from build123d import *

# Parameters (mm, degrees)
SKETCH1_W                    = 126
SKETCH1_H                    = 130
SKETCH1_R                    = 32.5
SKETCH1_W_2                  = 4.9
SKETCH1_H_2                  = 20
BOSS_EXTRUDE1_DEPTH          = 3
SKETCH2_W                    = 2.9
SKETCH2_H                    = 20
CUT_EXTRUDE1_DEPTH           = 3
F_4_0_4_DIAMETER_HOLE1_D     = 4
F_4_0_4_DIAMETER_HOLE1_DEPTH = 10
F_4_0_4_DIAMETER_HOLE1_TIP   = 1.201721238
SKETCH6_R                    = 2.3
CUT_EXTRUDE2_DEPTH           = 3


with BuildPart() as part:
    # Sketch1 → Boss-Extrude1 (new body)
    with BuildSketch(Plane.XY):
        with Locations((0, -5)):
            Rectangle(SKETCH1_W, SKETCH1_H)
        Circle(SKETCH1_R, mode=Mode.SUBTRACT)
        with Locations((-17.5, -54.9)):
            Rectangle(SKETCH1_W_2, SKETCH1_H_2, mode=Mode.SUBTRACT)
        with Locations((17.5, -54.9)):
            Rectangle(SKETCH1_W_2, SKETCH1_H_2, mode=Mode.SUBTRACT)
    extrude(amount=BOSS_EXTRUDE1_DEPTH)

    # Sketch2 → Cut-Extrude1 (cut)
    with BuildSketch(Plane.XY.offset(3)):
        with Locations((-56.5, -0.4)):
            Rectangle(SKETCH2_W, SKETCH2_H)
    cut_extrude1 = extrude(amount=-CUT_EXTRUDE1_DEPTH, mode=Mode.SUBTRACT)

    # Mirror1: Cut-Extrude1 across plane
    add(cut_extrude1.mirror(Plane(origin=(0, 0, 0), x_dir=(0, 0, 1), z_dir=(1, 0, 0))), mode=Mode.SUBTRACT)

    # Ø4.0 (4) Diameter Hole1
    with Locations(Plane.XY.offset(3)):
        with Locations((-24, 41.569219382), (48, 0), (24, 41.569219382), (24, -41.569219382), (-24, -41.569219382), (-48, 0)):
            Hole(F_4_0_4_DIAMETER_HOLE1_D / 2, depth=F_4_0_4_DIAMETER_HOLE1_DEPTH)
            with Locations((0, 0, -(F_4_0_4_DIAMETER_HOLE1_DEPTH + F_4_0_4_DIAMETER_HOLE1_TIP / 2))):  # 118° drill point
                Cone(0, F_4_0_4_DIAMETER_HOLE1_D / 2, F_4_0_4_DIAMETER_HOLE1_TIP, mode=Mode.SUBTRACT)

    # Sketch6 → Cut-Extrude2 (cut)
    with BuildSketch(Plane.XY.offset(3)):
        with Locations((0, -64)):
            Circle(SKETCH6_R)
    extrude(amount=-CUT_EXTRUDE2_DEPTH, mode=Mode.SUBTRACT)


solid = part.part
The listing builds one solid part. Answer for the finished solid, in the listing's coordinates (mm). A direction names the side the tool comes from. Round coordinates to 2 decimals unless told otherwise and drop trailing zeros. Write each loop counter-clockwise with the first axis right and the second up, starting at its lowest first coordinate (ties: lowest second). Pieces come first, ordered by that corner, then holes. Notation, with made-up numbers: M 17.25,60 L 31.25,60 A16 ccw 31.25,88 Z; hole C -27,37.25 d5. An arc over 180 degrees is marked long. Write each question's results on one line, items separated by ' | '. Start each with the question number.
Item 1: A cutting plane is placed at A-A on y = -53.5. Write down the section's boundary in (x, z).
Item 2: Straight lines are drawn through the part: L1, parallel to X at y = -52, z = 2.75; L2, parallel to Y at x = 0, z = 0.9; L3, parallel to X at y = -8, z = 0.8. For each, find the intervals that lie inside material, in ascending order. Write a range as [from, to].
Item 3: A flat-ended cylindrical pin translates along its axis: pin 1 Ø5.5 at (x, y) = (0, -64) entering from +Z. Find the tip coordinate at first contact, or state that the pin passes through.
Item 4: A cutting plane is placed at D-D on x = 24. Write down the section's boundary in (y, z).
Item 5: For faces 1 (the face through (-57.95, -1, 2)), 2 (the face through (63, -6, 1)), determine the directions among +Z, -Z, +X, -X, +Y, -Y from which every point of the face is accessible in a straight line to the end or side of a thin tool.
Item 6: A cutting plane is placed at C-C on y = -8. Write down the section's boundary in (x, z).
Item 7: A cutting plane is placed at B-B on x = -48. Write down the section's boundary in (y, z), and give its area (3 significant figures).
Item 8: For a pull along Y with two mould halves and no side action, classify faces 3 (the face through (17, -44.9, 1)), 4 (the face through (-1, 60, 1)), 5 (the face through (-1, -33, 3)) as pulls with the +Y half, pulls with the -Y half, needs draft (parallel to the pull), parting line crosses it, or undercut.
Check sheet entries:
1) outline: M -63,0 L -19.95,0 L -19.95,3 L -63,3 Z; M -15.05,0 L 15.05,0 L 15.05,3 L -15.05,3 Z; M 19.95,0 L 63,0 L 63,3 L 19.95,3 Z
2) L1: [-63, -19.95], [-15.05, 15.05], [19.95, 63] | L2: [-70, -66.3], [-61.7, -32.5], [32.5, 60] | L3: [-63, -57.95], [-55.05, -31.5], [31.5, 55.05], [57.95, 63]
3) pin 1: z = 3
4) outline: M -70,0 L -43.57,0 L -43.57,3 L -70,3 Z; M -39.57,0 L -21.91,0 L -21.91,3 L -39.57,3 Z; M 21.91,0 L 39.57,0 L 39.57,3 L 21.91,3 Z; M 43.57,0 L 60,0 L 60,3 L 43.57,3 Z
5) face 1: +Z, -Z | face 2: +Z, -Z, +X, +Y, -Y
6) outline: M -63,0 L -57.95,0 L -57.95,3 L -63,3 Z; M -55.05,0 L -31.5,0 L -31.5,3 L -55.05,3 Z; M 31.5,0 L 55.05,0 L 55.05,3 L 31.5,3 Z; M 57.95,0 L 63,0 L 63,3 L 57.95,3 Z
7) outline: M -70,0 L -2,0 L -2,3 L -70,3 Z; M 2,0 L 60,0 L 60,3 L 2,3 Z | area: 378 mm²
8) face 3: undercut | face 4: pulls with the +Y half | face 5: needs draft
